```python
from build123d import *

# Parameters (mm, degrees)
BASPROSKE_W         = 4.5
BASPROSKE_H         = 6.5
TOOTHCUT_DEPTH      = 11.234744745
TEETHCUTS_COUNT     = 24
TEETHCUTS_ANGLE     = 345
BORSKE_R            = 1.5
BORE_DEPTH          = 50.0000508
CUT_EXTRUDE_1_REACH = 13.408


with BuildPart() as part:
    # BasProSke → Base-Revolve (revolve)
    with BuildSketch(Plane(origin=(0, 0, 0), x_dir=(1, 0, 0), z_dir=(0, 1, 0)), mode=Mode.PRIVATE) as base_revolve_sk:
        with Locations((2.25, 3.25)):
            Rectangle(BASPROSKE_W, BASPROSKE_H)
    revolve(base_revolve_sk.sketch.rotate(Axis((-10, 0, 0), (1, 0, 0)), 180), axis=Axis((-10, 0, 0), (1, 0, 0)))

    # TooCutSke → ToothCut (cut, through all)
    with BuildSketch(Plane(origin=(0, 0, 0), x_dir=(0, 0, -1), z_dir=(1, 0, 0))):
        with BuildLine():
            ThreePointArc((0.241646108, 5.368564348), (0, 5.374), (-0.241646108, 5.368564348))
            ThreePointArc((-0.241646108, 5.368564348), (-0.413699957, 5.957993365), (-0.729686037, 6.48447403))
            ThreePointArc((-0.729686037, 6.48447403), (0, 6.5254), (0.729686037, 6.48447403))
            ThreePointArc((0.729686037, 6.48447403), (0.413699957, 5.957993365), (0.241646108, 5.368564348))
        make_face()
    toothcut = extrude(amount=TOOTHCUT_DEPTH, mode=Mode.SUBTRACT)

    # TeethCuts: ToothCut ×24 about axis
    teethcuts_axis = Axis((-10, 0, 0), (1, 0, 0))
    for i in range(1, TEETHCUTS_COUNT):
        add(toothcut.rotate(teethcuts_axis, i * TEETHCUTS_ANGLE / (TEETHCUTS_COUNT - 1)), mode=Mode.SUBTRACT)

    # BorSke → Bore (cut, symmetric)
    with BuildSketch(Plane(origin=(0, 0, 0), x_dir=(0, 0, -1), z_dir=(1, 0, 0))):
        with Locations(Location((0, 0, 0), (0, 0, 180))):
            Circle(BORSKE_R)
    extrude(amount=BORE_DEPTH, both=True, mode=Mode.SUBTRACT)

    # 草图1 → 旋转1 (revolve)
    with BuildSketch(Plane(origin=(0, 0, 0), x_dir=(1, 0, 0), z_dir=(0, 1, 0))):
        Polygon((0, 0), (-2.33, 0), (-2.33, 2.97), (0, 5.3), align=None)
    revolve(axis=Axis((0, 0, 0), (-1, 0, 0)))

    # 草图2 → 切除-拉伸1 (cut, up to next)
    with BuildSketch(Plane(origin=(4.5, 0, 0), x_dir=(0, 0, -1), z_dir=(1, 0, 0)), mode=Mode.PRIVATE) as cut_extrude_1_sk1:
        with BuildLine():
            Line((1.8, -0.871779789), (1.8, 0.871779789))
            ThreePointArc((1.8, 0.871779789), (-2, 0), (1.8, -0.871779789))
        make_face()
    cut_extrude_1_tool1 = extrude(cut_extrude_1_sk1.sketch, amount=-CUT_EXTRUDE_1_REACH, mode=Mode.PRIVATE) & part.part
    add(cut_extrude_1_tool1.solids().sort_by_distance((4.5, 0, 0.035819))[0], mode=Mode.SUBTRACT)


solid = part.part
```
Input: part model. Units: mm. Frame: model coordinates. A direction names the side the tool comes from. Round coordinates to 2 decimals unless told otherwise and drop trailing zeros. Loops run counter-clockwise (first coordinate to the right, second up) from the corner with the lowest first, then second, coordinate; pieces in that order, holes last.
1) Section query B-B on y = 0. Return the cut outline in (x, z), plus the area to 3 significant figures.
Ans:
outline: (-2.33, -2.97) - (0, -5.3) - (0, -5.37) - (4.5, -5.37) - (4.5, -1.8) - (-2.33, -1.8) - close; (-2.33, 2) - (4.5, 2) - (4.5, 5.37) - (0, 5.37) - (0, 5.3) - (-2.33, 2.97) - close
area: 41.7 mm2
2) Pull-direction query (Y, two-part tool) for faces 1 (the cylindrical face through (2.22, 5.95, -0.41)), 2 (the cylindrical face through (2.22, -5.36, -2.62)); classes: released by +Y, released by -Y, zero draft, split by the parting line, or undercut.
Ans:
face 1: released by +Y
face 2: undercut
3) Pin query (flat end, axial travel): pin 1 (1.5 mm diameter, centred on x = 3.5, y = 4.5, fed in from -Z); pin 2 (1 mm diameter, centred on x = 2.5, y = 2, fed in from -Z); pin 3 (4 mm diameter, centred on x = 0.5, z = -3.5, fed in from +Y); pin 4 (2.5 mm diameter, centred on y = 0, z = 0, fed in from -X). Return the tip coordinate at first contact, or that it passes through.
Ans:
pin 1: stops at z = -5.24
pin 2: stops at z = -6.06
pin 3: stops at y = 6.06
pin 4: passes through
4) Section query D-D on x = -0.5. Return the cut outline in (y, z).
Ans:
outline: circle Ø9.6 at (0, 0); hole (-0.87, -1.8) - (0.87, -1.8) arc R2 ccw (long way) to start
5) Material intervals for line 1 (Y direction, x = 2.75, z = 0); line 2 (Z direction, x = 2.5, y = -5), sorted ascending.
Ans:
line 1: y = -5.37 to -2, 2 to 5.37
line 2: z = -4.06 to -3.4, -2.55 to 2.55, 3.4 to 4.06
6) Section query C-C on y = 5.75. Return the cut outline in (x, z).
Ans:
outline: (0, -2.63) - (4.5, -2.63) - (4.5, -2.03) - (0, -2.03) - close; (0, -1.16) - (4.5, -1.16) - (4.5, -0.33) - (0, -0.33) - close; (0, 0.33) - (4.5, 0.33) - (4.5, 1.16) - (0, 1.16) - close; (0, 2.03) - (4.5, 2.03) - (4.5, 2.63) - (0, 2.63) - close
7) Set-up query: faces 3 (the cylindrical face through (2.218, -0.404, 5.937)), 4 (the cylindrical face through (2.218, 5.937, 0.404)), 5 (the cylindrical face through (2.22, 2.62, -5.36)). Return all of +Z, -Z, +X, -X, +Y, -Y with unobstructed straight access to the full face (end or side cutting, diameter ignored); none if empty.
Ans:
face 3: +Z, +X, -X
face 4: +X, -X, +Y
face 5: +X, -X
8) Section query A-A on z = 0. Return the cut outline in (x, y), plus the area to 3 significant figures.
Ans:
outline: (-2.33, -2.97) - (0, -5.3) - (0, -5.37) - (4.5, -5.37) - (4.5, -2) - (-2.33, -2) - close; (-2.33, 2) - (4.5, 2) - (4.5, 5.37) - (0, 5.37) - (0, 5.3) - (-2.33, 2.97) - close
area: 40.3 mm2
